```python
from build123d import *

# Parameters (mm, degrees)
SKETCH2_W           = 50
SKETCH2_H           = 33.5
SKETCH2_R           = 1.75
BOSS_EXTRUDE1_DEPTH = 8
BOSS_EXTRUDE2_DEPTH = 33.5
SKETCH6_R           = 1.75
CUT_EXTRUDE1_DEPTH  = 18.8


with BuildPart() as part:
    # Sketch2 → Boss-Extrude1 (new body)
    with BuildSketch(Plane.XY):
        Rectangle(SKETCH2_W, SKETCH2_H)
        with Locations((-20, 0)):
            Circle(SKETCH2_R, mode=Mode.SUBTRACT)
        with Locations((20, 0)):
            Circle(SKETCH2_R, mode=Mode.SUBTRACT)
    extrude(amount=BOSS_EXTRUDE1_DEPTH)

    # Sketch5 → Boss-Extrude2 (add)
    with BuildSketch(Plane.XZ.offset(16.75)):
        with BuildLine():
            Line((-25, 8), (-25, 17.8))
            Line((-25, 17.8), (-5.1, 17.8))
            Line((-5.1, 17.8), (-5.1, 8))
            Line((-5.1, 8), (5.1, 8))
            Line((5.1, 8), (5.1, 17.8))
            Line((5.1, 17.8), (25, 17.8))
            Line((25, 17.8), (25, 8))
            ThreePointArc((25, 8), (0, 0), (-25, 8))
        make_face()
    extrude(amount=-BOSS_EXTRUDE2_DEPTH)

    # Sketch6 → Cut-Extrude1 (cut, through all)
    with BuildSketch(Plane(origin=(0, 0, 0), x_dir=(-1, 0, 0), z_dir=(0, 0, -1))):
        with Locations((20, 0)):
            Circle(SKETCH6_R)
        with Locations((-20, 0)):
            Circle(SKETCH6_R)
    extrude(amount=-CUT_EXTRUDE1_DEPTH, mode=Mode.SUBTRACT)


solid = part.part
```
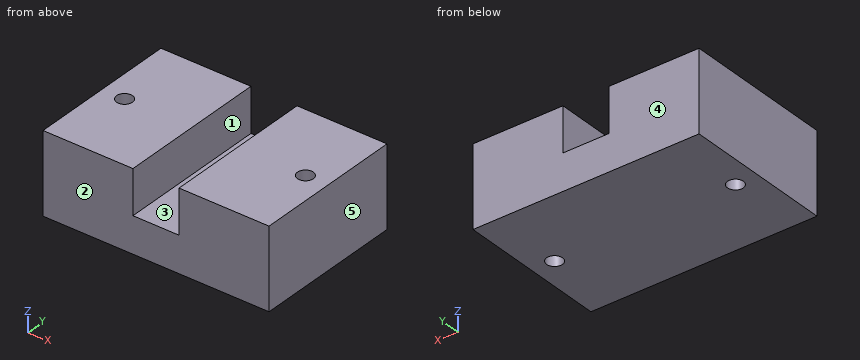
Model file for the job. Use its own axes, mm. Face numbers are marked on the shaded views. A direction names the side the tool comes from. Give positions to 0.01 mm unless a question says otherwise; leave off trailing zeros. Write each loop counter-clockwise with the first axis right and the second up, starting at its lowest first coordinate (ties: lowest second). Pieces come first, ordered by that corner, then holes. Notation, with made-up numbers: (1.5, 78) - (48.5, 78) arc R5 ccw to (48.5, 86) - close; hole circle Ø5 at (-28, -20.5). An arc over 180 degrees is marked (long way). One line per question, with ' | ' between items. Start each with the question number.
(1) Slice it at C-C on y = -6. Write the cut outline in (x, z).
(2) Slice it at B-B on x = 20. Write the cut outline in (y, z).
(3) Two-plate mould, pull along X, no slides. Class the marked faces 3, 4 and 5: +X half, -X half, draft (parallel to the pull), parting line (faces both ways), or undercut.
(4) 3-axis set-ups, long thin cutter, end or side, ignore diameter. For the marked faces 1 and 2: which of +Z, -Z, +X, -X, +Y, -Y reach the whole face in a straight line?
(5) Slice it at A-A on z = 15.75. Write the cut outline in (x, y).
(6) Wall check: line 1 along X through (y, z) = (0, 7.5); line 2 along Y through (x, z) = (-20, 4.45); line 3 along X through (y, z) = (-5.5, 14). Give the ranges that are in metal, low to high. Write a range as from..to.
(7) Pin check, flat tips, straight feed: P1, Ø5, axis at x = -2, y = -3.5, coming from the +Z side; P2, Ø6, axis at x = -2.5, y = 3, coming from the -Z side. Stop position of each tip, or through.
Results below:
1) outline: (-25, 0) - (25, 0) - (25, 17.8) - (5.1, 17.8) - (5.1, 8) - (-5.1, 8) - (-5.1, 17.8) - (-25, 17.8) - close
2) outline: (-16.75, 0) - (-1.75, 0) - (-1.75, 17.8) - (-16.75, 17.8) - close; (1.75, 0) - (16.75, 0) - (16.75, 17.8) - (1.75, 17.8) - close
3) face 3: undercut | face 4: draft | face 5: +X half
4) face 1: +Z, +Y, -Y | face 2: +Z, -Z, +X, -X, -Y
5) outline: (-25, -16.75) - (-5.1, -16.75) - (-5.1, 16.75) - (-25, 16.75) - close; (5.1, -16.75) - (25, -16.75) - (25, 16.75) - (5.1, 16.75) - close; hole circle Ø3.5 at (-20, 0); hole circle Ø3.5 at (20, 0)
6) line 1: -25..-21.75, -18.25..18.25, 21.75..25 | line 2: -16.75..-1.75, 1.75..16.75 | line 3: -25..-5.1, 5.1..25
7) P1: z = 8 | P2: z = 0
